Read the model definition and answer for the solid it produces. Units are mm, in the model's axes. Face numbers are marked on the shaded views. A direction names the side the tool comes from. Give positions to 0.01 mm unless a question says otherwise; leave off trailing zeros. Order: outer loops, then holes, each group sorted by start corner. A loop starts at its lowest first (then second) coordinate and runs counter-clockwise, first axis right, second up. Notation, with made-up numbers: M 56.25,-6 L 78.25,-6 A6 cw 78.25,0 Z; hole C 18,75 d1. An arc over 180 degrees is marked long. Write item = value, one per line. Start each with the question number.
from build123d import *

# Parameters (mm, degrees)
SKETCH_R        = 11.3
SKETCH_R_2      = 1.6
SKETCH_R_3      = 3.2
PAD_DEPTH       = 15
SKETCH001_R     = 3.2
POCKET_DEPTH    = 3.4
SKETCH002_R     = 6.1
POCKET001_DEPTH = 4


with BuildPart() as part:
    # Sketch → Pad (new body)
    with BuildSketch(Plane.XY):
        Polygon((20, 30), (20, 58), (62.3, 58), (62.3, 30), (82.3, 30), (82.3, 0), (0, 0), (0, 30), align=None)
        with Locations((41.15, 36.85)):
            Circle(SKETCH_R, mode=Mode.SUBTRACT)
        with Locations((25.65, 52.35)):
            Circle(SKETCH_R_2, mode=Mode.SUBTRACT)
        with Locations((25.65, 21.35)):
            Circle(SKETCH_R_2, mode=Mode.SUBTRACT)
        with Locations((56.65, 52.35)):
            Circle(SKETCH_R_2, mode=Mode.SUBTRACT)
        with Locations((56.65, 21.35)):
            Circle(SKETCH_R_2, mode=Mode.SUBTRACT)
        with Locations((11.15, 10)):
            Circle(SKETCH_R_3, mode=Mode.SUBTRACT)
        with Locations((31.15, 10)):
            Circle(SKETCH_R_3, mode=Mode.SUBTRACT)
        with Locations((51.15, 10)):
            Circle(SKETCH_R_3, mode=Mode.SUBTRACT)
        with Locations((71.15, 10)):
            Circle(SKETCH_R_3, mode=Mode.SUBTRACT)
    extrude(amount=PAD_DEPTH)

    # Sketch001 (on Face19 of Pad) → Pocket (cut)
    with BuildSketch(Plane.XY.offset(15)):
        with Locations((25.65, 52.35)):
            Circle(SKETCH001_R)
        with Locations((56.65, 52.35)):
            Circle(SKETCH001_R)
        with Locations((56.65, 21.35)):
            Circle(SKETCH001_R)
        with Locations((25.65, 21.35)):
            Circle(SKETCH001_R)
    extrude(amount=-POCKET_DEPTH, mode=Mode.SUBTRACT)

    # Sketch002 (on Face4 of Pocket) → Pocket001 (cut)
    with BuildSketch(Plane(origin=(0, 0, 0), x_dir=(1, 0, 0), z_dir=(0, 0, -1))):
        with Locations((11.15, -10)):
            Circle(SKETCH002_R)
        with Locations((31.15, -10)):
            Circle(SKETCH002_R)
        with Locations((51.15, -10)):
            Circle(SKETCH002_R)
        with Locations((71.15, -10)):
            Circle(SKETCH002_R)
    extrude(amount=-POCKET001_DEPTH, mode=Mode.SUBTRACT)


solid = part.part
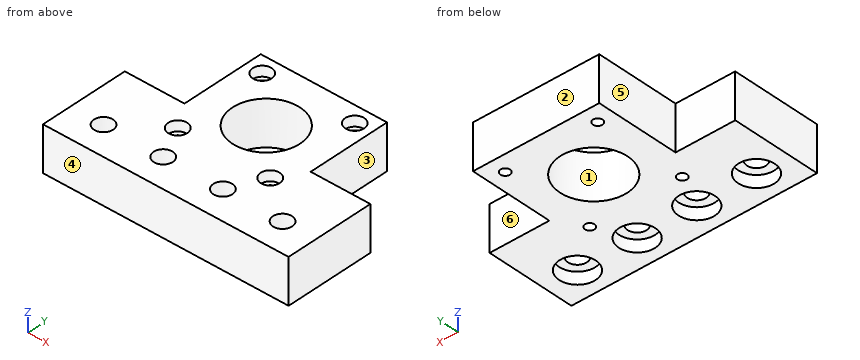
1) Find the intervals of material crossed by probe 1 along X at (y, z) = (52.35, 3); probe 2 along X at (y, z) = (10, 2.35); probe 3 along Y at (x, z) = (31.15, 10.25), in increasing order. Write a range as [from, to].
2) For the marked faces 4, 5 and 6, determine the directions among +Z, -Z, +X, -X, +Y, -Y from which every point of the face is accessible in a straight line to the end or side of a thin tool.
3) For a pull along Y with two mould halves and no side action, classify the marked faces 1, 2 and 3 as pulls with the +Y half, pulls with the -Y half, needs draft (parallel to the pull), parting line crosses it, or undercut.
4) Find section B-B on y = 21.35. Determine the outline of the cut face in (x, z).
5) Find section A-A on x = 71.15. Determine the outline of the cut face in (y, z), plus the area to 3 significant figures.
6) Each of these flat-tipped pins is pushed along its axis until it touches: P1, Ø7.5, axis at x = 31.15, y = 10, coming from the -Z side; P2, Ø7.5, axis at x = 69.5, z = 6, coming from the +Y side; P3, Ø6, axis at x = 71.15, y = 10, coming from the +Z side; P4, Ø1.9, axis at x = 26.5, y = 23, coming from the +Z side. Where does it stop, or does it pass through?
7) Find section C-C on z = 2.5. Count the separate pieces of the cut face and the enclosed holes in it, plus the area to 3 significant figures.
8) Find section D-D on x = 41.15. Determine the outline of the cut face in (y, z).
Numbers:
q1.probe_1 = [20, 24.05], [27.25, 55.05], [58.25, 62.3]
q1.probe_2 = [0, 5.05], [17.25, 25.05], [37.25, 45.05], [57.25, 65.05], [77.25, 82.3]
q1.probe_3 = [0, 6.8], [13.2, 31.59], [42.11, 58]
q2.face_4 = +Z, -Z, +X, -X, -Y
q2.face_5 = +Z, -Z, -X, +Y
q2.face_6 = +Z, -Z, +X, +Y
q3.face_1 = undercut
q3.face_2 = pulls with the +Y half
q3.face_3 = needs draft
q4.outline = M 0,0 L 24.05,0 L 24.05,11.6 L 22.45,11.6 L 22.45,15 L 0,15 Z; M 27.25,0 L 55.05,0 L 55.05,11.6 L 53.45,11.6 L 53.45,15 L 28.85,15 L 28.85,11.6 L 27.25,11.6 Z; M 58.25,0 L 82.3,0 L 82.3,15 L 59.85,15 L 59.85,11.6 L 58.25,11.6 Z
q5.outline = M 0,0 L 3.9,0 L 3.9,4 L 6.8,4 L 6.8,15 L 0,15 Z; M 13.2,4 L 16.1,4 L 16.1,0 L 30,0 L 30,15 L 13.2,15 Z
q5.area = 331 mm2
q6.P1 = 4
q6.P2 = 30
q6.P3 = through
q6.P4 = 11.6
q7.separate_pieces = 1
q7.enclosed_holes = 9
q7.area = 2,750 mm2
q8.outline = M 0,0 L 25.55,0 L 25.55,15 L 0,15 Z; M 48.15,0 L 58,0 L 58,15 L 48.15,15 Z
